```python
from build123d import *

# Parameters (mm, degrees)
FILLET1_R      = 0.4
CHAMFER1_SIZE  = 1
CHAMFER1_SIZE2 = 0.577350269


with BuildPart() as part:
    # Sketch1 → Revolve2 (revolve)
    with BuildSketch(Plane.XY):
        Polygon((0, 0), (0, 8.7), (-1.825, 8.7), (-1.825, 7), (-1.1, 7), (-1.1, 0), align=None)
    revolve(axis=Axis((0, 0, 0), (0, 1, 0)))

    # Fillet1
    fillet1_edges = [part.edges().sort_by_distance(p)[0] for p in [
        (1.825, 7, 0),
        (1.825, 8.7, 0),
    ]]
    fillet(fillet1_edges, radius=FILLET1_R)

    # Chamfer1
    chamfer1_edges = [part.edges().sort_by_distance(p)[0] for p in [
        (1.1, 0, 0),
    ]]
    chamfer1_side = [part.faces().sort_by_distance(p)[0] for p in [
        (1.1, 3.5, 0),
    ]]
    chamfer(chamfer1_edges, length=CHAMFER1_SIZE, length2=CHAMFER1_SIZE2, reference=chamfer1_side[0])


solid = part.part
```
Design review of the part built by this model. Coordinates are the model's own, in mm. A direction names the side the tool comes from. Coordinates: 2 decimals unless noted, no trailing zeros. Loops run counter-clockwise (first coordinate to the right, second up) from the corner with the lowest first, then second, coordinate; pieces in that order, holes last. Notation, with made-up numbers: (22, 41) - (73, 41) arc R21 ccw to (73, 48) - close; hole circle Ø4 at (45.5, 50.25). An arc over 180 degrees is marked (long way). Use CSV: the item, a comma, the result in double quotes. Start each with the question number.
1) Wall thickness on L1, parallel to Y at x = -1.25, z = -0.15; L2, parallel to Z at x = 0.05, y = 3.5; L3, parallel to Y at x = -0.65, z = -0.2: over which ranges is each line inside the solid? List them lowest first. Write a range as from..to.
2) Consider section C-C on y = 8. Write out the cut boundary in (x, z) (3 decimals).
3) For pin 1 Ø2 at (y, z) = (1, -1) entering from -X; pin 2 Ø1 at (x, y) = (-1, 4.5) entering from -Z, all flat-tipped, find the tip position at first contact; note any pin that passes through.
4) Tool access review of faces 1 (the flat face through (0, 0, 0)), 2 (the cylindrical face through (-1.05, 3.96, 0.33)): name each direction out of +Z, -Z, +X, -X, +Y, -Y from which nothing blocks a thin tool from reaching the whole face with its end or side.
5) Consider section D-D on y = 1.25. Write out the cut boundary in (x, z).
6) Consider section B-B on z = 0. Write out the cut boundary in (x, y) (3 decimals), then the cut area to 3 significant figures.
7) Consider section A-A on x = 0. Write out the cut boundary in (y, z) (3 decimals).
Geometry says:
1,L1,"7..8.7"
1,L2,"-1.1..1.1"
1,L3,"0.27..8.7"
2,outline,"circle Ø3.65 at (0, 0)"
3,pin 1,"x = -1.1"
3,pin 2,"z = -0.98"
4,face 1,"+Z, -Z, +X, -X, -Y"
4,face 2,"-Y"
5,outline,"circle Ø2.2 at (0, 0)"
6,outline,"(-1.825, 7.4) arc R0.4 ccw to (-1.425, 7) - (-1.1, 7) - (-1.1, 1) - (-0.523, 0) - (0.523, 0) - (1.1, 1) - (1.1, 7) - (1.425, 7) arc R0.4 ccw to (1.825, 7.4) - (1.825, 8.3) arc R0.4 ccw to (1.425, 8.7) - (-1.425, 8.7) arc R0.4 ccw to (-1.825, 8.3) - close"
6,area,"20.9 mm^2"
7,outline,"(0, -0.523) - (1, -1.1) - (7, -1.1) - (7, -1.425) arc R0.4 ccw to (7.4, -1.825) - (8.3, -1.825) arc R0.4 ccw to (8.7, -1.425) - (8.7, 1.425) arc R0.4 ccw to (8.3, 1.825) - (7.4, 1.825) arc R0.4 ccw to (7, 1.425) - (7, 1.1) - (1, 1.1) - (0, 0.523) - close"
